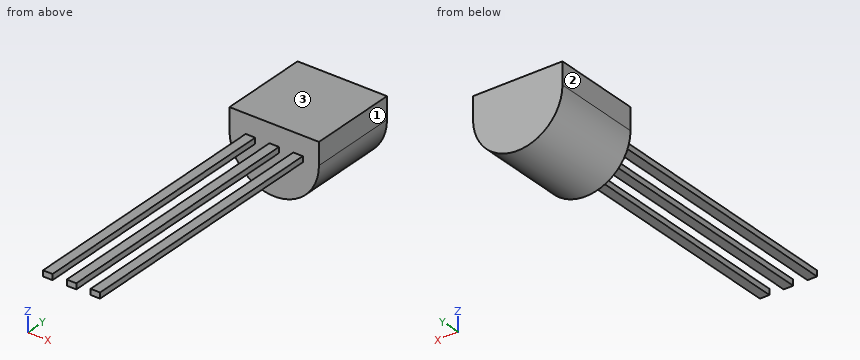
```python
from build123d import *

# Parameters (mm, degrees)
EXTRUDE_1_DEPTH = 4.7
SKETCH_2_W      = 0.5
SKETCH_2_H      = 0.3
EXTRUDE_2_DEPTH = 14


with BuildPart() as part:
    # 草图1 → 凸台-拉伸1 (new body)
    with BuildSketch(Plane(origin=(0, 0, 0), x_dir=(1, 0, 0), z_dir=(0, 1, 0))):
        with BuildLine():
            Line((-2.35, 0), (2.35, 0))
            Line((2.35, 0), (2.35, 1.15))
            ThreePointArc((2.35, 1.15), (0, 3.5), (-2.35, 1.15))
            Line((-2.35, 1.15), (-2.35, 0))
        make_face()
    extrude(amount=EXTRUDE_1_DEPTH)

    # 草图2 → 凸台-拉伸2 (add)
    with BuildSketch(Plane.XZ):
        with Locations((1.25, -1.15)):
            Rectangle(SKETCH_2_W, SKETCH_2_H)
        with Locations((0, -1.15)):
            Rectangle(SKETCH_2_W, SKETCH_2_H)
        with Locations((-1.25, -1.15)):
            Rectangle(SKETCH_2_W, SKETCH_2_H)
    extrude(amount=EXTRUDE_2_DEPTH)


solid = part.part
```
The listing builds one solid part. Answer for the finished solid, in the listing's coordinates (mm). Face numbers are marked on the shaded views. Coordinates: 2 decimals unless noted, no trailing zeros. Write each loop counter-clockwise with the first axis right and the second up, starting at its lowest first coordinate (ties: lowest second). Pieces come first, ordered by that corner, then holes. Notation, with made-up numbers: (28.5, -7.5) - (54.5, -7.5) arc R31 ccw to (54.5, 26.5) - close; hole circle Ø1 at (58.5, 69.5). An arc over 180 degrees is marked (long way). Return JSON: item names as keys, results as strings. Group by question number.
Q1. The part is cut by section A-A on y = -1. Write down the section's boundary in (x, z).
Q2. Flat-ended cylindrical pins translate along their axes: pin 1 Ø0.6 at (x, y) = (-1, -6) entering from +Z; pin 2 Ø2 at (x, y) = (-1, -3) entering from -Z. Find the tip coordinate at first contact, or state that the pin passes through.
Q3. The part is cut by section B-B on x = 0. Write down the section's boundary in (y, z).
Q4. Find the intervals of material crossed by line 1 along Y through (x, z) = (1.55, -0.4); line 2 along Z through (x, y) = (-0.05, -9.75); line 3 along Z through (x, y) = (-0.4, 3), in increasing order. Write a range as [from, to].
Q5. For a pull along X with two mould halves and no side action, classify the marked faces 1, 2 and 3 as +X half, -X half, draft (parallel to the pull), parting line (faces both ways), or undercut.
Q6. The part is cut by section C-C on z = -0.5. Write down the section's boundary in (x, y), and give its area (3 significant figures).
Q7. The part is cut by section D-D on z = -2.25. Write down the section's boundary in (x, y).
Evaluation:
{
 "1": {"outline": "(-1.5, -1.3) - (-1, -1.3) - (-1, -1) - (-1.5, -1) - close; (-0.25, -1.3) - (0.25, -1.3) - (0.25, -1) - (-0.25, -1) - close; (1, -1.3) - (1.5, -1.3) - (1.5, -1) - (1, -1) - close"},
 "2": {"pin 1": "stops at z = -1", "pin 2": "stops at z = -1.3"},
 "3": {"outline": "(-14, -1.3) - (0, -1.3) - (0, -3.5) - (4.7, -3.5) - (4.7, 0) - (0, 0) - (0, -1) - (-14, -1) - close"},
 "4": {"line 1": "y = [0, 4.7]", "line 2": "z = [-1.3, -1]", "line 3": "z = [-3.47, 0]"},
 "5": {"face 1": "+X half", "face 2": "-X half", "face 3": "draft"},
 "6": {"outline": "(-2.35, 0) - (2.35, 0) - (2.35, 4.7) - (-2.35, 4.7) - close", "area": "22.1 mm2"},
 "7": {"outline": "(-2.08, 0) - (2.08, 0) - (2.08, 4.7) - (-2.08, 4.7) - close"}
}
